Can you work these out from the model? Positions are in its coordinate system, mm. A direction names the side the tool comes from. Give positions to 0.01 mm unless a question says otherwise; leave off trailing zeros. Order: outer loops, then holes, each group sorted by start corner. A loop starts at its lowest first (then second) coordinate and runs counter-clockwise, first axis right, second up. Notation, with made-up numbers: M 68,-29.5 L 112,-29.5 A23 cw 112,9.5 Z; hole C 60.25,23.5 d4. An arc over 180 degrees is marked long. Use one line per item in the form item = value. Start each with the question number.
1. I want a section at C-C, the plane x = 11. List the corners of the cut face in (y, z) for me, and give its area (3 significant figures).
2. I want a section at A-A, the plane x = 0. List the corners of the cut face in (y, z) for me, and give its area (3 significant figures).
3. For faces 4 (the face through (-5, 0, 20.825)), 5 (the face through (-25.5, 0, 26)), 6 (the face through (-0.74, -3.32, -25.41)), 7 (the face through (5, 0, -19)), which set-ups out of +Z, -Z, +X, -X, +Y, -Y let a thin tool reach every point of the face, with its end or its side?
4. I need wall thicknesses on L1, parallel to Z at x = -8.5, y = -3.5; L2, parallel to Y at x = 0, z = -23.75; L3, parallel to Z at x = 18, y = 0.5. Which ranges of each line are inside material? Lowest first, please.
5. I want a section at B-B, the plane y = 0. List the corners of the cut face in (x, z) for me, and give its area (3 significant figures).
6. We'd pull the mould along Y, two halves only. Please class faces 1 (the face through (-0.74, -3.32, 26.33)), 2 (the face through (-6, 0, 16.825)), 3 (the face through (0, -6.35, 0)): +Y half, -Y half, draft (parallel to the pull), parting line (faces both ways), or undercut.
7. I want a section at D-D, the plane x = 17.5. List the corners of the cut face in (y, z) for me, and give its area (3 significant figures).
8. Will this pin go through, and if not, where does the flat tip stop? P1, Ø5.5, axis at x = 0, y = 0, coming from the +Z side.
```python
from build123d import *

# Parameters (mm, degrees)
SKETCH_1_W               = 51
SKETCH_1_H               = 64
EXTRUDE_1_DEPTH          = 6.35
CUT_EXTRUDE_1_DEPTH      = 43.843202495
PATTERN_CIRCULAR_1_COUNT = 2
HOLE_WIZARD_M8_1_D       = 6.8
HOLE_WIZARD_M8_1_DEPTH   = 13


with BuildPart() as part:
    # 草图1 → 凸台-拉伸1 (new, symmetric)
    with BuildSketch(Plane(origin=(0, 0, 0), x_dir=(1, 0, 0), z_dir=(0, 1, 0))):
        Rectangle(SKETCH_1_W, SKETCH_1_H)
    extrude(amount=EXTRUDE_1_DEPTH, both=True)

    # 草图2 → 切除-拉伸1 (cut, through all)
    with BuildSketch(Plane(origin=(0, 6.35, 0), x_dir=(1, 0, 0), z_dir=(0, 1, 0))):
        with BuildLine():
            Line((25.5, 15), (-14.5, 15))
            ThreePointArc((-14.5, 15), (-16.5, 17), (-14.5, 19))
            Line((-14.5, 19), (25.5, 19))
            ThreePointArc((25.5, 19), (27.5, 17), (25.5, 15))
        make_face()
    cut_extrude_1 = extrude(amount=-CUT_EXTRUDE_1_DEPTH, mode=Mode.SUBTRACT)

    # 阵列(圆周)1: 切除-拉伸1 ×2 about axis
    pattern_circular_1_axis = Axis((-0.252947744, 0, 0.912547634), (0, 1, 0))
    for i in range(1, PATTERN_CIRCULAR_1_COUNT):
        add(cut_extrude_1.rotate(pattern_circular_1_axis, i * 360 / PATTERN_CIRCULAR_1_COUNT), mode=Mode.SUBTRACT)

    # M8 螺纹孔1
    with Locations(Plane(origin=(0, 0, -32), x_dir=(-1, 0, 0), z_dir=(0, 0, -1))):
        with Locations((0, 0)):
            hole_wizard_m8_1 = Hole(HOLE_WIZARD_M8_1_D / 2, depth=HOLE_WIZARD_M8_1_DEPTH)

    # 镜向1: M8 螺纹孔1 across plane
    add(hole_wizard_m8_1.mirror(Plane.XY), mode=Mode.SUBTRACT)


solid = part.part
```
Check result:
q1.outline = M -6.35,-32 L 6.35,-32 L 6.35,-19 L -6.35,-19 Z; M -6.35,-15 L 6.35,-15 L 6.35,16.83 L -6.35,16.83 Z; M -6.35,20.83 L 6.35,20.83 L 6.35,32 L -6.35,32 Z
q1.area = 711 mm2
q2.outline = M -6.35,-32 L -3.4,-32 L -3.4,-19 L -6.35,-19 Z; M -6.35,-15 L 6.35,-15 L 6.35,16.83 L -6.35,16.83 Z; M -6.35,20.83 L -3.4,20.83 L -3.4,32 L -6.35,32 Z; M 3.4,-32 L 6.35,-32 L 6.35,-19 L 3.4,-19 Z; M 3.4,20.83 L 6.35,20.83 L 6.35,32 L 3.4,32 Z
q2.area = 547 mm2
q3.face_4 = -X, +Y, -Y
q3.face_5 = +Z, -Z, -X, +Y, -Y
q3.face_6 = -Z
q3.face_7 = +X, +Y, -Y
q4.L1 = -32 to -19, -15 to 16.83, 20.83 to 32
q4.L2 = -6.35 to -3.4, 3.4 to 6.35
q4.L3 = -32 to -19, -15 to 32
q5.outline = M -25.5,-32 L -3.4,-32 L -3.4,-19 L -14.5,-19 A2 cw -14.5,-15 L 25.5,-15 L 25.5,32 L 3.4,32 L 3.4,20.83 L 13.99,20.83 A2 cw 13.99,16.83 L -25.5,16.83 Z; M -25.5,20.83 L -3.4,20.83 L -3.4,32 L -25.5,32 Z; M 3.4,-32 L 25.5,-32 L 25.5,-19 L 3.4,-19 Z
q5.area = 2,770 mm2
q6.face_1 = undercut
q6.face_2 = draft
q6.face_3 = -Y half
q7.outline = M -6.35,-32 L 6.35,-32 L 6.35,-19 L -6.35,-19 Z; M -6.35,-15 L 6.35,-15 L 6.35,32 L -6.35,32 Z
q7.area = 762 mm2
q8.P1 = 16.83
